from build123d import *

# Parameters (mm, degrees)
SKETCH_1_R          = 10
EXTRUDE_1_DEPTH     = 20
SKETCH_2_R          = 12.5
EXTRUDE_2_DEPTH     = 15
SKETCH_3_R          = 15
EXTRUDE_3_DEPTH     = 60
SKETCH_4_R          = 12.5
EXTRUDE_4_DEPTH     = 15
SKETCH_5_R          = 11
EXTRUDE_5_DEPTH     = 5
SKETCH_6_W          = 15
SKETCH_6_H          = 15
EXTRUDE_6_DEPTH     = 35
SKETCH_7_R          = 3
CUT_EXTRUDE_1_DEPTH = 20
SKETCH_8_R          = 2
CUT_EXTRUDE_2_DEPTH = 20
SKETCH_9_W          = 35
SKETCH_9_H          = 10.5
CUT_EXTRUDE_3_DEPTH = 20
SKETCH_10_R         = 3.5
CUT_EXTRUDE_4_DEPTH = 20
FILLET_1_R          = 1


with BuildPart() as part:
    # 草图1 → 凸台-拉伸1 (new body)
    with BuildSketch(Plane.XY):
        Circle(SKETCH_1_R)
    extrude(amount=EXTRUDE_1_DEPTH)

    # 草图2 → 凸台-拉伸2 (add)
    with BuildSketch(Plane.XY.offset(20)):
        Circle(SKETCH_2_R)
    extrude(amount=EXTRUDE_2_DEPTH)

    # 草图3 → 凸台-拉伸3 (add)
    with BuildSketch(Plane.XY.offset(35)):
        Circle(SKETCH_3_R)
    extrude(amount=EXTRUDE_3_DEPTH)

    # 草图4 → 凸台-拉伸4 (add)
    with BuildSketch(Plane.XY.offset(95)):
        Circle(SKETCH_4_R)
    extrude(amount=EXTRUDE_4_DEPTH)

    # 草图5 → 凸台-拉伸5 (add)
    with BuildSketch(Plane.XY.offset(110)):
        Circle(SKETCH_5_R)
    extrude(amount=EXTRUDE_5_DEPTH)

    # 草图6 → 凸台-拉伸6 (add)
    with BuildSketch(Plane.XY.offset(115)):
        Rectangle(SKETCH_6_W, SKETCH_6_H)
    extrude(amount=EXTRUDE_6_DEPTH)

    # 草图7 → 切除-拉伸1 (cut)
    with BuildSketch(Plane(origin=(0, 0, 0), x_dir=(-1, 0, 0), z_dir=(0, 0, -1))):
        Circle(SKETCH_7_R)
    extrude(amount=-CUT_EXTRUDE_1_DEPTH, mode=Mode.SUBTRACT)

    # 草图8 → 切除-拉伸2 (cut, symmetric)
    with BuildSketch(Plane(origin=(0, 0, 0), x_dir=(0, 0, -1), z_dir=(1, 0, 0))):
        with Locations((-7, 0)):
            Circle(SKETCH_8_R)
    extrude(amount=CUT_EXTRUDE_2_DEPTH, both=True, mode=Mode.SUBTRACT)

    # 草图9 → 切除-拉伸3 (cut, symmetric)
    with BuildSketch(Plane(origin=(0, 0, 0), x_dir=(0, 0, -1), z_dir=(1, 0, 0))):
        with Locations((-65, -9.75)):
            Rectangle(SKETCH_9_W, SKETCH_9_H)
    extrude(amount=CUT_EXTRUDE_3_DEPTH, both=True, mode=Mode.SUBTRACT)

    # 草图10 → 切除-拉伸4 (cut, symmetric)
    with BuildSketch(Plane(origin=(0, 0, 0), x_dir=(0, 0, -1), z_dir=(1, 0, 0))):
        with Locations((-142, 0)):
            Circle(SKETCH_10_R)
        with Locations((-123, 0)):
            Circle(SKETCH_10_R)
    extrude(amount=CUT_EXTRUDE_4_DEPTH, both=True, mode=Mode.SUBTRACT)

    # 圆角1
    fillet_1_edges = [part.edges().sort_by_distance(p)[0] for p in [
        (-7.5, 7.5, 132.5),
        (-7.5, -7.5, 132.5),
        (7.5, -7.5, 132.5),
        (7.5, 7.5, 132.5),
    ]]
    fillet(fillet_1_edges, radius=FILLET_1_R)


solid = part.part
Geometry: final body of the model. Coordinates: model frame, mm. A direction names the side the tool comes from. Give positions to 0.01 mm unless a question says otherwise; leave off trailing zeros. Write each loop counter-clockwise with the first axis right and the second up, starting at its lowest first coordinate (ties: lowest second). Pieces come first, ordered by that corner, then holes.
(1) Mould query, pull axis Y, two halves, no side actions, for faces 1 (the flat face through (-3.4, 12.3, 95)), 2 (the cylindrical face through (6, 2, 7)), 3 (the cylindrical face through (0.105, -1.341, 119.767)), 4 (the cylindrical face through (-2.38, -10.74, 112.46)). Classes: released by +Y, released by -Y, zero draft, split by the parting line, or undercut.
(2) Access query for faces 5 (the cylindrical face through (2.21, 2.03, 9.86)), 6 (the flat face through (0, -9, 82.5)), 7 (the flat face through (0, 7.5, 132)). Directions: +Z, -Z, +X, -X, +Y, -Y. A direction counts if a zero-diameter tool reaches every point of the face in a straight line with its end or side. Return the directions, or none.
(3) Cut plane B-B, the plane x = 0. Give the number of separate pieces and of enclosed holes in the cut face, then the cut area to 3 significant figures.
(4) Cut plane D-D, the plane z = 7. Return loops of the section in (x, y), then the cut area to 3 significant figures.
(5) Cut plane A-A, the plane z = 142. Return loops of the section in (x, y).
(6) Ray query, line 1 (Y direction, x = -1, z = 142); line 2 (Y direction, x = 0, z = 5.5); line 3 (Z direction, x = 8.25, y = -11.5). Return the intervals inside material, ascending.
(7) First-contact query: P1, Ø4, axis at x = 3.5, z = 38, coming from the +Y side; P2, Ø6.5, axis at y = -1, z = 126.5, coming from the -X side; P3, Ø6, axis at x = -5.5, z = 53, coming from the -Y side. Flat tips, straight axial feed; report the tip coordinate or a pass-through.
Values follow:
1. face 1: zero draft
1. face 2: undercut
1. face 3: undercut
1. face 4: split by the parting line
2. face 5: -Z
2. face 6: +X, -X, -Y
2. face 7: +Z, +X, -X, +Y
3. separate pieces: 1
3. enclosed holes: 2
3. area: 3,020 mm2
4. outline: (-9.8, -2) arc R10 ccw to (9.8, -2) - (2.24, -2) arc R3 cw to (-2.24, -2) - close; (-9.8, 2) - (-2.24, 2) arc R3 cw to (2.24, 2) - (9.8, 2) arc R10 ccw to start
4. area: 229 mm2
5. outline: (-7.5, -6.5) arc R1 ccw to (-6.5, -7.5) - (6.5, -7.5) arc R1 ccw to (7.5, -6.5) - (7.5, -3.5) - (-7.5, -3.5) - close; (-7.5, 3.5) - (7.5, 3.5) - (7.5, 6.5) arc R1 ccw to (6.5, 7.5) - (-6.5, 7.5) arc R1 ccw to (-7.5, 6.5) - close
6. line 1: y = -7.5 to -3.5, 3.5 to 7.5
6. line 2: y = -10 to -3, 3 to 10
6. line 3: z = 35 to 47.5, 82.5 to 95
7. P1: stops at y = 14.92
7. P2: stops at x = -7.5
7. P3: stops at y = -4.5
